Work out the finished part from the listing and answer in its coordinate system (mm). Coordinates: 2 decimals unless noted, no trailing zeros. Loops run counter-clockwise (first coordinate to the right, second up) from the corner with the lowest first, then second, coordinate; pieces in that order, holes last.
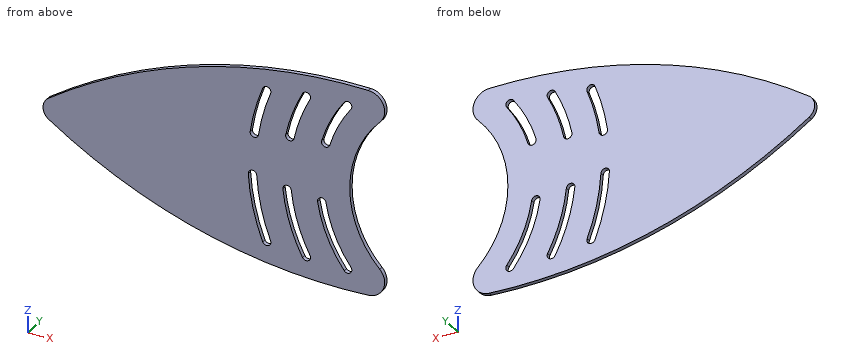
```python
from build123d import *

# Parameters (mm, degrees)
F1_DEPTH = 3.175


# Not quite as in the source:
# - ends of sketch curves that miss each other by under 0.0002 mm in the source are joined


with BuildPart() as f1:
    # F0 (on Front) → F1 (new body)
    with BuildSketch(Plane.XZ):
        with BuildLine():
            ThreePointArc((-123.4070797919, 1.8233010265), (-127.5387969828, -6.0085300089), (-123.4070915827, -13.8403672647))
            ThreePointArc((-123.4070915827, -13.8403672647), (-9.7633198011, -67.3185862363), (114.9359014402, -82.3162835053))
            ThreePointArc((114.9359014402, -82.3162835053), (126.1869378761, -74.3359779231), (123.456379114, -60.815058194))
            ThreePointArc((123.456379114, -60.815058194), (101.0612030172, -6.0085281204), (123.4563821883, 48.798006178))
            ThreePointArc((123.4563821883, 48.798006178), (126.1869343608, 62.3189124907), (114.9359007509, 70.2992174423))
            ThreePointArc((114.9359007509, 70.2992174423), (-9.7633198011, 55.3015372363), (-123.4070797919, 1.8233010265))
        make_face()
        with BuildLine():
            ThreePointArc((77.0821397385, -22.5154604101), (79.7004591586, -18.8888761314), (83.3270330978, -21.5072098724))
            ThreePointArc((83.3270330978, -21.5072098724), (89.9643653266, -44.3549576844), (101.9514625839, -64.9069229437))
            ThreePointArc((101.9514625839, -64.9069229437), (101.3506333254, -69.3393586044), (96.9181875419, -68.7385326678))
            ThreePointArc((96.9181875419, -68.7385326678), (84.1512609661, -46.8495678563), (77.0821397385, -22.5154604101))
        make_face(mode=Mode.SUBTRACT)
        with BuildLine():
            ThreePointArc((25.4272095012, -15.2152278243), (28.3955581041, -11.8691050411), (31.7416808873, -14.837453644))
            ThreePointArc((31.7416808873, -14.837453644), (35.0399400748, -38.2666108744), (42.033430024, -60.8695978255))
            ThreePointArc((42.033430024, -60.8695978255), (40.2700359641, -64.9803081743), (36.1593147519, -63.2169312407))
            ThreePointArc((36.1593147519, -63.2169312407), (28.8665917441, -39.6468400601), (25.4272095012, -15.2152278243))
        make_face(mode=Mode.SUBTRACT)
        with BuildLine():
            ThreePointArc((51.2038323174, -19.8796162989), (54.0078974535, -16.3946587115), (57.4928438898, -19.1987377064))
            ThreePointArc((57.4928438898, -19.1987377064), (62.2856351867, -42.3239729178), (71.4255090517, -64.1003387977))
            ThreePointArc((71.4255090517, -64.1003387977), (70.1400475431, -68.384628042), (65.855751892, -67.099154634))
            ThreePointArc((65.855751892, -67.099154634), (56.24403894, -44.1986400904), (51.2038323174, -19.8796162989))
        make_face(mode=Mode.SUBTRACT)
        with BuildLine():
            ThreePointArc((26.8321292417, 16.6896378099), (30.4920693109, 34.2160200507), (36.1593192267, 51.1998804526))
            ThreePointArc((36.1593192267, 51.1998804526), (40.2700359641, 52.9632591743), (42.0334342681, 48.8525471295))
            ThreePointArc((42.0334342681, 48.8525471295), (36.5987212677, 32.5655461507), (33.0889530651, 15.7582851057))
            ThreePointArc((33.0889530651, 15.7582851057), (29.4948750618, 13.0955480188), (26.8321292417, 16.6896378099))
        make_face(mode=Mode.SUBTRACT)
        with BuildLine():
            ThreePointArc((53.3645508696, 21.2199967221), (58.4187785321, 38.5905299983), (65.8557505543, 55.0821063543))
            ThreePointArc((65.8557505543, 55.0821063543), (70.1400475431, 56.367579042), (71.425520951, 52.0832833909))
            ThreePointArc((71.425520951, 52.0832833909), (64.3536192611, 36.4012543788), (59.5474961242, 19.8834151887))
            ThreePointArc((59.5474961242, 19.8834151887), (55.7877392052, 17.4602445799), (53.3645508696, 21.2199967221))
        make_face(mode=Mode.SUBTRACT)
        with BuildLine():
            ThreePointArc((80.1169824074, 23.7207222996), (87.030580802, 40.9781600378), (96.9181889515, 56.7214825948))
            ThreePointArc((96.9181889515, 56.7214825948), (101.3506333254, 57.3223096044), (101.9514733693, 52.8898657333))
            ThreePointArc((101.9514733693, 52.8898657333), (92.6678111275, 38.108160652), (86.1765020812, 21.9048248522))
            ThreePointArc((86.1765020812, 21.9048248522), (82.2387981181, 19.7830123613), (80.1169824074, 23.7207222996))
        make_face(mode=Mode.SUBTRACT)
    extrude(amount=F1_DEPTH)


solid = f1.part
```
1. A cutting plane is placed at A-A, the plane y = -1.05. Count the separate pieces of the cut face and the enclosed holes in it, then the cut area to 3 significant figures.
2. A cutting plane is placed at D-D, the plane x = -17. Give the vertices of the cut face in (y, z) (3 decimals).
3. A cutting plane is placed at B-B, the plane z = -42. Give the vertices of the cut face in (x, y) (3 decimals).
4. A cutting plane is placed at C-C, the plane x = -88. Give the vertices of the cut face in (y, z) (3 decimals).
5. Straight lines are drawn through the part: probe 1 along X at (y, z) = (-2.05, -22); probe 2 along X at (y, z) = (-0.55, -20); probe 3 along X at (y, z) = (-1.15, 19). For each, find the intervals that lie inside material, in ascending order.
Answers below:
1. separate pieces: 1
1. enclosed holes: 6
1. area: 24,600 mm2
2. outline: (-3.175, -65.164) - (0, -65.164) - (0, 53.147) - (-3.175, 53.147) - close
3. outline: (-75.24, -3.175) - (29.412, -3.175) - (29.412, 0) - (-75.24, 0) - close; (35.926, -3.175) - (55.583, -3.175) - (55.583, 0) - (35.926, 0) - close; (62.186, -3.175) - (82.213, -3.175) - (82.213, 0) - (62.186, 0) - close; (88.99, -3.175) - (109.828, -3.175) - (109.828, 0) - (88.99, 0) - close
4. outline: (-3.175, -35.415) - (0, -35.415) - (0, 23.398) - (-3.175, 23.398) - close
5. probe 1: x = -110.98 to 25.98, 32.35 to 51.45, 57.83 to 77.04, 83.41 to 102.71
5. probe 2: x = -114.12 to 25.79, 32.14 to 51.22, 57.58 to 77.76, 82.65 to 102.32
5. probe 3: x = -95.94 to 27.19, 33.61 to 53.7, 59.21 to 105.16
